from build123d import *

# Parameters (mm, degrees)
SKETCH1_W               = 25
SKETCH1_H               = 25
BOSS_EXTRUDE1_DEPTH     = 7
BOSS_EXTRUDE2_DEPTH     = 15.2
SKETCH3_W               = 25
SKETCH3_H               = 25
BOSS_EXTRUDE3_DEPTH     = 6
CUT_EXTRUDE1_DEPTH      = 28.603260677
CUT_EXTRUDE1_DEPTH_BACK = 28.603260677
SKETCH4_R               = 1.425
SKETCH5_R               = 2.5
SKETCH5_R_2             = 1.425
BOSS_EXTRUDE4_DEPTH     = 1.5
BOSS_EXTRUDE5_START     = 1.5
SKETCH6_R               = 2.5
SKETCH6_R_2             = 1.425
BOSS_EXTRUDE5_DEPTH     = 1.5
FILLET1_R               = 3
CHAMFER2_SIZE           = 0.25
CHAMFER3_SIZE           = 0.5
SKETCH8_W               = 7
SKETCH8_H               = 25
SKETCH8_R               = 1.6
BOSS_EXTRUDE6_DEPTH     = 7


with BuildPart() as part:
    # Sketch1 → Boss-Extrude1 (new body)
    with BuildSketch(Plane(origin=(0, 0, 0), x_dir=(1, 0, 0), z_dir=(0, 1, 0))):
        Rectangle(SKETCH1_W, SKETCH1_H)
    extrude(amount=BOSS_EXTRUDE1_DEPTH)

    # Sketch2 → Boss-Extrude2 (add)
    with BuildSketch(Plane(origin=(0, 7, 0), x_dir=(1, 0, 0), z_dir=(0, 1, 0))):
        Polygon((-12.5, -12.5), (-7.897681384, -12.5), (-7.897681384, 8.291292288), (12.5, 8.291292288), (12.5, 12.5), (-12.5, 12.5), align=None)
    extrude(amount=BOSS_EXTRUDE2_DEPTH)

    # Sketch3 → Boss-Extrude3 (add)
    with BuildSketch(Plane(origin=(0, 22.2, 0), x_dir=(1, 0, 0), z_dir=(0, 1, 0))):
        Rectangle(SKETCH3_W, SKETCH3_H)
    extrude(amount=BOSS_EXTRUDE3_DEPTH)

    # Sketch4 → Cut-Extrude1 (cut, two sides: drawn at the far end of the back side and taken through both)
    with BuildSketch(Plane(origin=(0, 7, 0), x_dir=(1, 0, 0), z_dir=(0, 1, 0)).offset(-CUT_EXTRUDE1_DEPTH_BACK)):
        with Locations(Location((2.301159308, -2.104353856, 0), (0, 0, 270))):
            Circle(SKETCH4_R)
    extrude(amount=CUT_EXTRUDE1_DEPTH + CUT_EXTRUDE1_DEPTH_BACK, mode=Mode.SUBTRACT)

    # Sketch5 → Boss-Extrude4 (add)
    with BuildSketch(Plane(origin=(0, 7, 0), x_dir=(1, 0, 0), z_dir=(0, 1, 0))):
        with Locations(Location((2.301159308, -2.104353856, 0), (0, 0, 90))):
            Circle(SKETCH5_R)
        with Locations(Location((2.301159308, -2.104353856, 0), (0, 0, 270))):
            Circle(SKETCH5_R_2, mode=Mode.SUBTRACT)
    extrude(amount=BOSS_EXTRUDE4_DEPTH)

    # Sketch6 → Boss-Extrude5 (add)
    with BuildSketch(Plane.XZ.offset(-22.2).offset(BOSS_EXTRUDE5_START)):
        with Locations(Location((2.301159308, 2.104353856, 0), (0, 0, 270))):
            Circle(SKETCH6_R)
        with Locations(Location((2.301159308, 2.104353856, 0), (0, 0, 90))):
            Circle(SKETCH6_R_2, mode=Mode.SUBTRACT)
    extrude(amount=-BOSS_EXTRUDE5_DEPTH)

    # Fillet1
    # the kernel refuses this fillet: 3 mm, written as the material it adds along each edge
    with BuildSketch(Plane(origin=(2.301159308, 7, 2.104353856), x_dir=(0, 0, -1), z_dir=(1, 0, 0))) as fillet1_piece_1:
        with BuildLine():
            CenterArc((5.098076211, 3), FILLET1_R, 210, 60)
            Line((2.5, 1.5), (2.448038476, 1.47))
            ThreePointArc((2.448038476, 1.47), (2.44, 0.75), (2.44, 0))
            Line((2.44, 0), (2.5, -0.06))
            Line((2.5, -0.06), (5.098076211, -0.06))
            Line((5.098076211, -0.06), (5.098076211, 0))
        make_face()
    revolve(axis=Axis((2.301159308, 7, 2.104353856), (0, 1, 0)))
    with BuildSketch(Plane(origin=(2.301159308, 22.2, 2.104353856), x_dir=(0, 0, -1), z_dir=(-1, 0, 0))) as fillet1_piece_2:
        with BuildLine():
            CenterArc((5.098076211, 3), FILLET1_R, 210, 60)
            Line((2.5, 1.5), (2.448038476, 1.47))
            ThreePointArc((2.448038476, 1.47), (2.44, 0.75), (2.44, 0))
            Line((2.44, 0), (2.5, -0.06))
            Line((2.5, -0.06), (5.098076211, -0.06))
            Line((5.098076211, -0.06), (5.098076211, 0))
        make_face()
    revolve(axis=Axis((2.301159308, 22.2, 2.104353856), (0, -1, 0)))

    # Chamfer1
    # the kernel refuses this chamfer: 1, 0.396795558 mm, written as the material it takes off along each edge
    with BuildSketch(Plane(origin=(2.301159308, 8.5, 2.104353856), x_dir=(0, 0, -1), z_dir=(1, 0, 0))) as chamfer1_piece_1:
        with BuildLine():
            Line((2.245190561, 0.026572252), (3.029375179, -0.670372697))
            Line((3.029375179, -0.670372697), (3.043365842, -0.656080694))
            ThreePointArc((3.043365842, -0.656080694), (2.755730305, -0.342231162), (2.517320508, 0.01))
            Line((2.517320508, 0.01), (2.5, 0.02))
            ThreePointArc((2.5, 0.02), (2.37259528, 0.02), (2.245190561, 0.046572252))
            Line((2.245190561, 0.046572252), (2.245190561, 0.026572252))
        make_face()
    revolve(axis=Axis((2.301159308, 8.5, 2.104353856), (0, 1, 0)), mode=Mode.SUBTRACT)
    with BuildSketch(Plane(origin=(2.301159308, 20.7, 2.104353856), x_dir=(0, 0, -1), z_dir=(-1, 0, 0))) as chamfer1_piece_2:
        with BuildLine():
            Line((3.029375179, -0.670372697), (2.245190561, 0.026572252))
            Line((2.245190561, 0.026572252), (2.245190561, 0.046572252))
            ThreePointArc((2.245190561, 0.046572252), (2.37259528, 0.02), (2.5, 0.02))
            Line((2.5, 0.02), (2.517320508, 0.01))
            ThreePointArc((2.517320508, 0.01), (2.755730305, -0.342231162), (3.043365842, -0.656080694))
            Line((3.043365842, -0.656080694), (3.029375179, -0.670372697))
        make_face()
    revolve(axis=Axis((2.301159308, 20.7, 2.104353856), (0, -1, 0)), mode=Mode.SUBTRACT)

    # Chamfer2
    chamfer2_edges = [part.edges().sort_by_distance(p)[0] for p in [
        (2.301159308, 8.5, 0.679353856),
        (2.301159308, 20.7, 0.679353856),
    ]]
    chamfer(chamfer2_edges, length=CHAMFER2_SIZE)

    # Chamfer3
    chamfer3_edges = [part.edges().sort_by_distance(p)[0] for p in [
        (2.301159308, 0, 0.679353856),
        (2.301159308, 28.2, 0.679353856),
    ]]
    chamfer(chamfer3_edges, length=CHAMFER3_SIZE)

    # Sketch8 → Boss-Extrude6 (add)
    # profile 1 of 2: a face of its own
    with BuildSketch(Plane(origin=(0, 0, 0), x_dir=(1, 0, 0), z_dir=(0, 1, 0))):
        with Locations((16, 0)):
            Rectangle(SKETCH8_W, SKETCH8_H)
        with Locations(Location((16, -2.104353856, 0), (0, 0, 90))):
            Circle(SKETCH8_R, mode=Mode.SUBTRACT)
    # profile 2 of 2: a face of its own
    with BuildSketch(Plane(origin=(0, 0, 0), x_dir=(1, 0, 0), z_dir=(0, 1, 0))):
        with Locations((-16, 0)):
            Rectangle(SKETCH8_W, SKETCH8_H)
        with Locations(Location((-16, -2.104353856, 0), (0, 0, 90))):
            Circle(SKETCH8_R, mode=Mode.SUBTRACT)
    extrude(amount=BOSS_EXTRUDE6_DEPTH)


solid = part.part
Work out the finished part from the listing and answer in its coordinate system (mm). A direction names the side the tool comes from. Give positions to 0.01 mm unless a question says otherwise; leave off trailing zeros. Write each loop counter-clockwise with the first axis right and the second up, starting at its lowest first coordinate (ties: lowest second). Pieces come first, ordered by that corner, then holes. Notation, with made-up numbers: (-7, -18) - (42, -18) arc R28 cw to (42, 19) - close; hole circle Ø4 at (88.5, 62.25). An arc over 180 degrees is marked (long way). One line per item, written item: value. Start each with the question number.
1. Find section A-A (x = -7). Write down the section's boundary in (y, z).
2. Consider probe 1 along Y at (x, z) = (4, 9.5); probe 2 along Z at (x, y) = (-16, 3.5); probe 3 along X at (y, z) = (1.5, 3.25). Determine where each line is inside the solid, lowest interval first.
3. For faces 1 (the flat face through (-2.4, 22.2, -0.4)), 2 (the flat face through (4, 8.5, 3)), 3 (the flat face through (0, 0, 0)), determine the directions among +Z, -Z, +X, -X, +Y, -Y from which every point of the face is accessible in a straight line to the end or side of a thin tool.
4. Find section C-C (z = -7.75). Write down the section's boundary in (x, y).
5. Given pin 1 (12 mm diameter, centred on x = 4.5, y = 15, fed in from +Z); pin 2 (6.5 mm diameter, centred on y = 20.5, z = 1, fed in from +X); pin 3 (12 mm diameter, centred on y = 14.5, z = 4.5, fed in from -X), each flat-ended and moving along its own axis, determine where each tip first touches the part or whether it passes through.
6. Find section B-B (x = -16). Write down the section's boundary in (y, z), then the cut area to 3 significant figures.
7. Find section D-D (y = 10.5). Write down the section's boundary in (x, z).
8. For a pull along Z with two mould halves and no side action, classify faces 4 (the cylindrical face through (14.414, 3.451, 2.313)), 5 (the flat face through (0, 5, 12.5)), 6 (the flat face through (-16, 7, 0)) as +Z half, -Z half, draft (parallel to the pull), parting line (faces both ways), or undercut.
Geometry results:
1. outline: (0, -12.5) - (28.2, -12.5) - (28.2, 12.5) - (22.2, 12.5) - (22.2, -8.29) - (7, -8.29) - (7, 12.5) - (0, 12.5) - close
2. probe 1: 0 to 7, 22.2 to 28.2
2. probe 2: -12.5 to 0.5, 3.7 to 12.5
2. probe 3: -19.5 to -17.12, -14.88 to 1.45, 3.15 to 14.88, 17.12 to 19.5
3. face 1: none
3. face 2: +Z, +X
3. face 3: +Z, -Z, +X, -X, -Y
4. outline: (-19.5, 0) - (19.5, 0) - (19.5, 7) - (-7.9, 7) - (-7.9, 22.2) - (12.5, 22.2) - (12.5, 28.2) - (-12.5, 28.2) - (-12.5, 7) - (-19.5, 7) - close
5. pin 1: z = 4.4
5. pin 2: x = 12.5
5. pin 3: x = -12.5
6. outline: (0, -12.5) - (7, -12.5) - (7, 0.5) - (0, 0.5) - close; (0, 3.7) - (7, 3.7) - (7, 12.5) - (0, 12.5) - close
6. area: 153 mm2
7. outline: (-12.5, -12.5) - (12.5, -12.5) - (12.5, -8.29) - (-7.9, -8.29) - (-7.9, 12.5) - (-12.5, 12.5) - close
8. face 4: undercut
8. face 5: +Z half
8. face 6: draft
